Build history of the part. All positions in model axes, mm. Round coordinates to 2 decimals unless told otherwise and drop trailing zeros. Loops run counter-clockwise (first coordinate to the right, second up) from the corner with the lowest first, then second, coordinate; pieces in that order, holes last. Notation, with made-up numbers: M -35.5,16.5 L 21.5,16.5 A25 cw 21.5,33.5 Z; hole C 7,85 d1. An arc over 180 degrees is marked long. Use one line per item in the form item = value. Start each with the question number.
Autodesk Inventor part; units mm, degrees
ref_plane "YZ Plane" through (0, 0, 0) normal (1, 0, 0) x (0, 1, 0)
ref_plane "XZ Plane" through (0, 0, 0) normal (0, 1, 0) x (-1, 0, 0)
ref_plane "XY Plane" through (0, 0, 0) normal (0, 0, 1) x (1, 0, 0)
sketch "Sketch1" plane through (0, 0, 0) normal (0, 1, 0) x (-1, 0, 0)
  circle A0 centre (0, 0) radius 5
  dimension "d0" = 10
extrude "Extrusion1" add sketch "Sketch1" along normal blind 800
sketch "Sketch2" plane through (0, 800, 0) normal (0, 1, 0) x (1, 0, 0)
  point P0 (0, 0)
  point P1 (0, 0)
hole "Hole1" at (0, 800, 0) direction (0, -1, 0) diameter 3.242 depth 12 tip angle 118
chamfer "Chamfer1" distance 0.5 angle 45 3 edges at (0, 800, -1.621) (5, 800, 0) (5, 0, 0)
properties part number "CUT_ALU_10x800mm_Rod"
Q1. Wall check: probe 1 along Z at (x, y) = (0, 793.75); probe 2 along X at (y, z) = (681, 0.75); probe 3 along X at (y, z) = (644, 0.5). Give the ranges that are in metal, low to high.
Q2. Saw through at A-A (y = 218.5). Give the cut face in (x, z), and give its area (3 significant figures).
Q3. Drop a flat-ended pin along its axis: P1, Ø1.5, axis at x = 3, y = 657, coming from the -Z side. Give the stop position or say it passes through.
Filled in:
q1.probe_1 = -5 to -1.62, 1.62 to 5
q1.probe_2 = -4.94 to 4.94
q1.probe_3 = -4.97 to 4.97
q2.outline = C 0,0 d10
q2.area = 78.5 mm²
q3.P1 = -4.47
